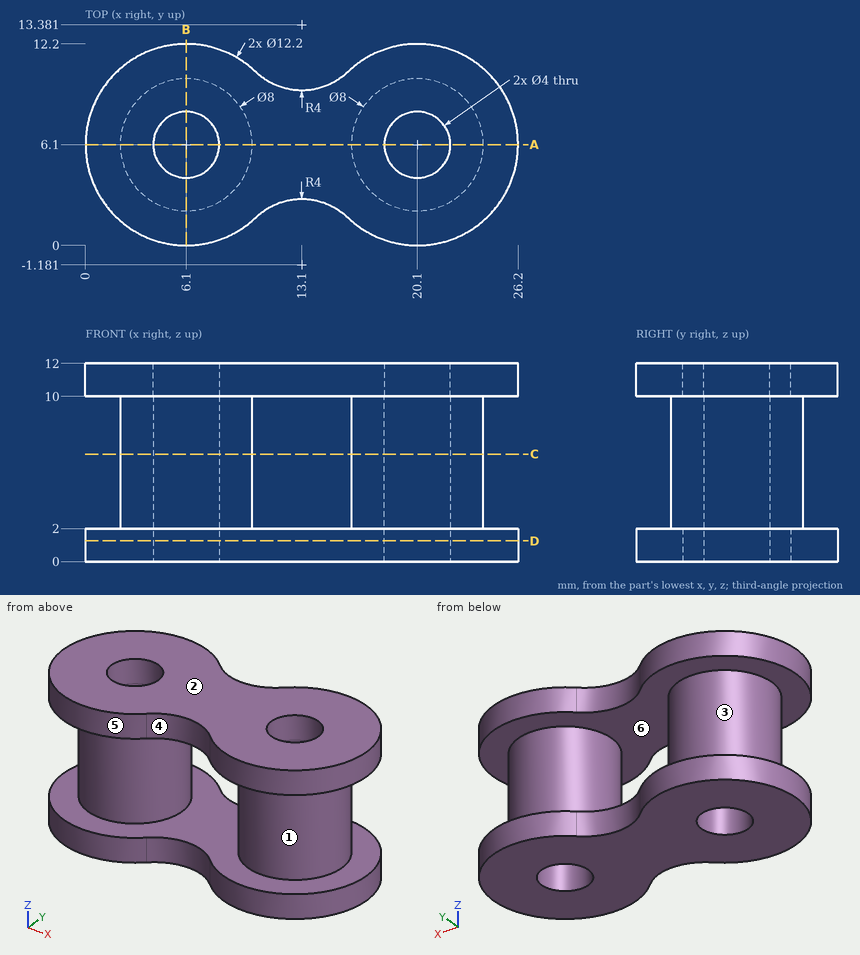
Geometry: see drawing. Coordinates: mm, zero at the bounding-box minimum. A direction names the side the tool comes from. Round coordinates to 2 decimals unless told otherwise and drop trailing zeros. Write each loop counter-clockwise with the first axis right and the second up, starting at its lowest first coordinate (ties: lowest second). Pieces come first, ordered by that corner, then holes.
Item 1: Section query C-C (z = 6.5). Return loops of the section in (x, y).
Item 2: Pin query (flat end, axial travel): P1, Ø2, axis at x = 15.5, z = 10, coming from the +Y side (1 decimal); P2, Ø2.5, axis at x = 20.1, y = 6.1, coming from the -Z side; P3, Ø1.5, axis at y = 2.5, z = 1, coming from the +X side; P4, Ø3, axis at y = 9.5, z = 4, coming from the -X side. Return the tip coordinate at first contact, or that it passes through.
Item 3: Set-up query: the marked faces 5 and 6. Return all of +Z, -Z, +X, -X, +Y, -Y with unobstructed straight access to the full face (end or side cutting, diameter ignored); none if empty.
Item 4: Mould query, pull axis Z, two halves, no side actions, for the marked faces 1, 2, 3 and 4. Classes: +Z half, -Z half, draft (parallel to the pull), parting line (faces both ways), or undercut.
Item 5: Section query D-D (z = 1.25). Return loops of the section in (x, y), plus the area to 3 significant figures.
Item 6: Material intervals for L1, parallel to X at y = 6.1, z = 5.75; L2, parallel to Y at x = 20.1, z = 10.95; L3, parallel to X at y = 6.1, z = 11.45, sorted ascending.
Item 7: Section query B-B (x = 6.1). Return loops of the section in (y, z), plus the area to 3 significant figures.
Item 8: Section query A-A (y = 6.1). Return loops of the section in (x, z), plus the area to 3 significant figures.
Completed:
1. outline: circle Ø8 at (6.1, 6.1); circle Ø8 at (20.1, 6.1); hole circle Ø4 at (6.1, 6.1); hole circle Ø4 at (20.1, 6.1)
2. P1: stops at y = 11
2. P2: passes through
2. P3: stops at x = 25.49
2. P4: stops at x = 2.58
3. face 5: +Z, -Z
3. face 6: none
4. face 1: undercut
4. face 2: +Z half
4. face 3: undercut
4. face 4: draft
5. outline: (10.33, 1.7) arc R4 cw to (15.87, 1.7) arc R6.1 ccw (long way) to (15.87, 10.5) arc R4 cw to (10.33, 10.5) arc R6.1 ccw (long way) to start; hole circle Ø4 at (6.1, 6.1); hole circle Ø4 at (20.1, 6.1)
5. area: 226 mm2
6. L1: x = 2.1 to 4.1, 8.1 to 10.1, 16.1 to 18.1, 22.1 to 24.1
6. L2: y = 0 to 4.1, 8.1 to 12.2
6. L3: x = 0 to 4.1, 8.1 to 18.1, 22.1 to 26.2
7. outline: (0, 0) - (4.1, 0) - (4.1, 12) - (0, 12) - (0, 10) - (2.1, 10) - (2.1, 2) - (0, 2) - close; (8.1, 0) - (12.2, 0) - (12.2, 2) - (10.1, 2) - (10.1, 10) - (12.2, 10) - (12.2, 12) - (8.1, 12) - close
7. area: 64.8 mm2
8. outline: (0, 0) - (4.1, 0) - (4.1, 12) - (0, 12) - (0, 10) - (2.1, 10) - (2.1, 2) - (0, 2) - close; (8.1, 0) - (18.1, 0) - (18.1, 12) - (8.1, 12) - close; (22.1, 0) - (26.2, 0) - (26.2, 2) - (24.1, 2) - (24.1, 10) - (26.2, 10) - (26.2, 12) - (22.1, 12) - close; hole (10.1, 2) - (16.1, 2) - (16.1, 10) - (10.1, 10) - close
8. area: 137 mm2
